Check sheet for the modelled part. Datum: model origin and axes. Units: mm. A direction names the side the tool comes from. Coordinates: 2 decimals unless noted, no trailing zeros. Loops run counter-clockwise (first coordinate to the right, second up) from the corner with the lowest first, then second, coordinate; pieces in that order, holes last. Notation, with made-up numbers: (-9.5, -31.75) -> (35.5, -31.75) arc R13 cw to (35.5, -26.75) -> close; hole circle Ø3 at (-28.5, 39.5). An arc over 180 degrees is marked (long way). Use CSV: the item, a comma, the result in double quotes. Start each with the question number.
1. Release check for a two-part mould opening along X. For faces 4 (the face through (4.366, -6, 23)), 5 (the face through (6.91, -1.45, 33.4)), 6 (the face through (33.4, -1.45, 6.98)) record: pulls with the +X half, pulls with the -X half, needs draft (parallel to the pull), parting line crosses it, or undercut.
2. Set-up check for faces 1 (the face through (23, -6, 4.366)), 2 (the face through (-4.366, -6, 23)), 3 (the face through (21, -8, 9.525)): record each of +Z, -Z, +X, -X, +Y, -Y from which the full face is reachable in a straight line by a thin tool's end or side.
3. Sectioned sample at C-C, the plane z = 21.5. Record the cut outline in (x, y) (3 decimals), and give its area (3 significant figures).
4. Sectioned sample at A-A, the plane x = 25.4. Record the cut outline in (y, z) (1 decimal).
5. Thickness scan on L1, parallel to Z at x = 27, y = -5.75 (3 decimals); L2, parallel to Y at x = 6.2, z = 25.4 (1 decimal). Record the ranges inside material, lowest first.
6. Sectioned sample at B-B, the plane z = -8.5. Record the cut outline in (x, y) (1 decimal), and give its area (3 significant figures).
7. Gauge pin test, flat ends, axial feed: pin 1 (4 mm diameter, centred on x = 28, y = -9.5, fed in from +Z) (3 decimals); pin 2 (8 mm diameter, centred on y = -9, z = 20.5, fed in from -X) (3 decimals); pin 3 (4 mm diameter, centred on x = -9, y = -4.5, fed in from -Z); pin 4 (4 mm diameter, centred on x = 25.4, y = -7.94, fed in from +Z). Record the tip position at first contact, or that the pin passes through.
8. Sectioned sample at D-D, the plane x = 0. Record the cut outline in (y, z) (3 decimals).
```python
from build123d import *

# Parameters (mm, degrees)
F0_R     = 15.875
F0_R_2   = 11.1379
F1_DEPTH = 15.875
F3_DEPTH = 15.875
F4_R     = 11.1379
F5_DEPTH = 15.876
F6_R     = 2.5
F7_DEPTH = 25.401
F9_DEPTH = 44.451
F10_R    = 5.08


with BuildPart() as f1:
    # F0 (on Front) → F1 (new body)
    with BuildSketch(Plane.XZ):
        Circle(F0_R)
        Circle(F0_R_2, mode=Mode.SUBTRACT)
    extrude(amount=F1_DEPTH)

    # F2 (on face) → F3 (join, through all)
    with BuildSketch(Plane.XZ.offset(15.875)):
        with BuildLine():
            Line((-4.365625, 15.875), (-4.365625, 34.925))
            Line((-4.365625, 34.925), (-9.525, 34.925))
            Line((-9.525, 34.925), (-9.525, 12.7))
            ThreePointArc((-9.525, 12.7), (-5.0201157855, 15.0603473566), (0, 15.875))
            Line((0, 15.875), (-4.365625, 15.875))
        make_face()
        with BuildLine():
            Line((9.525, 12.7), (9.525, 34.925))
            Line((9.525, 34.925), (4.365625, 34.925))
            Line((4.365625, 34.925), (4.365625, 15.875))
            Line((4.365625, 15.875), (0, 15.875))
            ThreePointArc((0, 15.875), (5.0201157855, 15.0603473566), (9.525, 12.7))
        make_face()
        with BuildLine():
            Line((34.925, 9.525), (12.7, 9.525))
            ThreePointArc((12.7, 9.525), (15.0603473566, 5.0201157855), (15.875, 0))
            Line((15.875, 0), (15.875, 4.365625))
            Line((15.875, 4.365625), (34.925, 4.365625))
            Line((34.925, 4.365625), (34.925, 9.525))
        make_face()
        with BuildLine():
            Line((15.875, -4.365625), (15.875, 0))
            ThreePointArc((15.875, 0), (15.0603473566, -5.0201157855), (12.7, -9.525))
            Line((12.7, -9.525), (34.925, -9.525))
            Line((34.925, -9.525), (34.925, -4.365625))
            Line((34.925, -4.365625), (15.875, -4.365625))
        make_face()
    extrude(amount=-F3_DEPTH)

    # F4 (on Front) → F5 (cut, through all)
    with BuildSketch(Plane.XZ):
        Circle(F4_R)
    extrude(amount=F5_DEPTH, mode=Mode.SUBTRACT)

    # F6 (on face) → F7 (cut, through all)
    with BuildSketch(Plane.XY.offset(9.525)):
        with Locations((25.4, -7.9375)):
            Circle(F6_R)
    extrude(amount=-F7_DEPTH, mode=Mode.SUBTRACT)

    # F8 (on face) → F9 (cut, through all)
    with BuildSketch(Plane(origin=(-9.525, 0, 0), x_dir=(0, -1, 0), z_dir=(-1, 0, 0))):
        with BuildLine():
            ThreePointArc((7.9375, 27.9), (6.169733047, 23.632233047), (10.4375, 25.4))
            ThreePointArc((10.4375, 25.4), (9.705266953, 27.167766953), (7.9375, 27.9))
        make_face()
    extrude(amount=-F9_DEPTH, mode=Mode.SUBTRACT)

    # F10
    f10_edges = [f1.edges().sort_by_distance(p)[0] for p in [
        (-6.945312, 0, 34.925),
        (6.945312, 0, 34.925),
        (6.945312, -15.875, 34.925),
        (-6.945312, -15.875, 34.925),
        (34.925, 0, 6.945312),
        (34.925, 0, -6.945312),
        (34.925, -15.875, 6.945312),
        (34.925, -15.875, -6.945312),
    ]]
    fillet(f10_edges, radius=F10_R)


solid = f1.part
```
Completed:
1,face 4,"undercut"
1,face 5,"needs draft"
1,face 6,"pulls with the +X half"
2,face 1,"+X, +Y, -Y"
2,face 2,"+Z, +Y, -Y"
2,face 3,"+Z, +X, +Y, -Y"
3,outline,"(-9.525, -15.875) -> (-4.366, -15.875) -> (-4.366, 0) -> (-9.525, 0) -> close; (4.366, -15.875) -> (9.525, -15.875) -> (9.525, 0) -> (4.366, 0) -> close"
3,area,"164 mm²"
4,outline,"(-15.9, -9.5) -> (-10.4, -9.5) -> (-10.4, -4.4) -> (-15.9, -4.4) -> close; (-15.9, 4.4) -> (-10.4, 4.4) -> (-10.4, 9.5) -> (-15.9, 9.5) -> close; (-5.4, -9.5) -> (0, -9.5) -> (0, -4.4) -> (-5.4, -4.4) -> close; (-5.4, 4.4) -> (0, 4.4) -> (0, 9.5) -> (-5.4, 9.5) -> close"
5,L1,"-9.525 to -4.366, 4.366 to 9.525"
5,L2,"-15.9 to -10.4, -5.4 to 0"
6,outline,"(-13.4, -15.9) -> (-7.2, -15.9) -> (-7.2, 0) -> (-13.4, 0) -> close; (7.2, -15.9) -> (29.8, -15.9) arc R5.1 ccw to (34.9, -10.8) -> (34.9, -5.1) arc R5.1 ccw to (29.8, 0) -> (7.2, 0) -> close; hole circle Ø5 at (25.4, -7.9)"
6,area,"508 mm²"
7,pin 1,"z = 9.525"
7,pin 2,"x = -9.525"
7,pin 3,"z = -14.25"
7,pin 4,"through"
8,outline,"(-15.875, -15.875) -> (0, -15.875) -> (0, -11.138) -> (-15.875, -11.138) -> close; (-15.875, 11.138) -> (0, 11.138) -> (0, 15.875) -> (-15.875, 15.875) -> close"
